```python
from build123d import *

# Parameters (mm, degrees)
CUT_EXTRUDE1_START = -4.2
CUT_EXTRUDE1_DEPTH = 4.2
CIRPATTERN1_COUNT  = 8
FILLET1_R          = 0.2


with BuildPart() as part:
    # Sketch1 → Revolve1 (revolve)
    with BuildSketch(Plane(origin=(0, 0, 0), x_dir=(0, 0, -1), z_dir=(1, 0, 0)), mode=Mode.PRIVATE) as revolve1_sk:
        with BuildLine():
            Line((0, 14.6), (0, 16.25))
            Line((0, 16.25), (0.3, 16.25))
            Line((0.3, 16.25), (0.3, 18.6))
            Line((0.3, 18.6), (0, 18.6))
            Line((0, 18.6), (0, 19.818460969))
            Line((0, 19.818460969), (1.2, 20.14))
            Line((1.2, 20.14), (5, 20.14))
            Line((5, 20.14), (6, 19.872050808))
            Line((6, 19.872050808), (6, 18.25))
            Line((6, 18.25), (5.5, 18.25))
            Line((5.5, 18.25), (5.5, 17.75))
            Line((5.5, 17.75), (2.4, 17.75))
            ThreePointArc((2.4, 17.75), (2.117157288, 17.632842712), (2, 17.35))
            Line((2, 17.35), (2, 15.2))
            Line((2, 15.2), (2.3, 15.2))
            ThreePointArc((2.3, 15.2), (3.249937225, 16.198746073), (4.294987437, 15.3))
            Line((4.294987437, 15.3), (4.5, 15.3))
            Line((4.5, 15.3), (4.5, 14.3))
            Line((4.5, 14.3), (3.297700441, 13.5))
            Line((3.297700441, 13.5), (1.3, 14.15))
            Line((1.3, 14.15), (-0.2, 13.85))
            Line((-0.2, 13.85), (-0.5, 13.85))
            Line((-0.5, 13.85), (-0.5, 14.25))
            Line((-0.5, 14.25), (0, 14.6))
        make_face()
    revolve(revolve1_sk.sketch.rotate(Axis((0, 0, 0), (0, 0, -1)), 90), axis=Axis((0, 0, 0), (0, 0, -1)))

    # Sketch3 → Cut-Extrude1 (cut)
    with BuildSketch(Plane(origin=(0, 0, -6), x_dir=(-1, 0, 0), z_dir=(0, 0, -1)).offset(CUT_EXTRUDE1_START)):
        with BuildLine():
            Line((-18.207141456, -1.25), (-16.3, -1.25))
            Line((-16.3, -1.25), (-16.3, 1.25))
            Line((-16.3, 1.25), (-18.207141456, 1.25))
            ThreePointArc((-18.207141456, 1.25), (-18.25, 0), (-18.207141456, -1.25))
        make_face()
    cut_extrude1 = extrude(amount=CUT_EXTRUDE1_DEPTH, mode=Mode.SUBTRACT)

    # CirPattern1: Cut-Extrude1 ×8 about axis
    cirpattern1_axis = Axis((0, 0, 0), (0, 0, 1))
    for i in range(1, CIRPATTERN1_COUNT):
        add(cut_extrude1.rotate(cirpattern1_axis, i * 360 / CIRPATTERN1_COUNT), mode=Mode.SUBTRACT)

    # Fillet1
    fillet1_edges = [part.edges().sort_by_distance(p)[0] for p in [
        (-19.872050808, 0, -6),
        (-19.818460969, 0, 0),
    ]]
    fillet(fillet1_edges, radius=FILLET1_R)


solid = part.part
```
Geometry: final body of the model. Coordinates: model frame, mm. A direction names the side the tool comes from. Give positions to 0.01 mm unless a question says otherwise; leave off trailing zeros. Return JSON: item names as keys, results as strings.
Item 1: Access query for faces 1 (the flat face through (0.1, 16.4, -0.3)), 2 (the flat face through (-11.76, -13.53, -3.37)). Directions: +Z, -Z, +X, -X, +Y, -Y. A direction counts if a zero-diameter tool reaches every point of the face in a straight line with its end or side. Return the directions, or none.
Filled in:
{"face 1": "+Z", "face 2": "-Z"}
Item 2: Mould query, pull axis X, two halves, no side actions, for faces 3 (the cylindrical face through (19.21, -6.05, -3.13)), 4 (the flat face through (11.76, 13.53, -3.37)), 5 (the flat face through (-17.4, 7.2, 0)). Classes: released by +X, released by -X, zero draft, split by the parting line, or undercut.
Filled in:
{"face 3": "split by the parting line", "face 4": "undercut", "face 5": "zero draft"}
Item 3: Pin query (flat end, axial travel): P1, Ø1.4, axis at x = -15.5, y = -4.5, coming from the -Z side; P2, Ø1, axis at x = 17.5, z = -4.5, coming from the +Y side; P3, Ø2, axis at x = -17.5, z = -3, coming from the -Y side. Return the tip coordinate at first contact, or that it passes through.
Filled in:
{"P1": "z = -4.27", "P2": "y = 10.8", "P3": "y = -11.55"}
Item 4: Line query: line 1 (X direction, y = -10, z = -4) (3 decimals); line 2 (X direction, y = 8, z = -3.5); line 3 (X direction, y = -14, z = -3.75). Output: solid intervals per line, ascending.
Filled in:
{"line 1": "-17.482 to -14.665, -12.38 to -9.751, 9.751 to 12.38, 14.665 to 17.482", "line 2": "-18.48 to -15.84, -14.06 to -11.04, 11.04 to 14.06, 15.84 to 18.48", "line 3": "-14.48 to -10.91, -7.94 to 7.94, 10.91 to 14.48"}
